```python
from build123d import *

# Parameters (mm, degrees)
EXTRUDE_1_DEPTH     = 4
EXTRUDE_START       = -2
SKETCH_2_R          = 0.75
EXTRUDE_2_DEPTH     = 1
SKETCH_3_R          = 0.75
CUT_EXTRUDE_1_DEPTH = 0.1
SKETCH_4_R          = 0.3
EXTRUDE_3_DEPTH     = 1.75


with BuildPart() as part:
    # 草图1 → 凸台-拉伸1 (new body)
    with BuildSketch(Plane.XY):
        with BuildLine():
            Line((0, 2), (9.3, 2))
            ThreePointArc((9.3, 2), (11.3, 0), (9.3, -2))
            Line((9.3, -2), (0, -2))
            ThreePointArc((0, -2), (-2, 0), (0, 2))
        make_face()
    extrude(amount=EXTRUDE_1_DEPTH)

    # 草图2 → 凸台-拉伸2 (add)
    with BuildSketch(Plane(origin=(0, 0, 0), x_dir=(-1, 0, 0), z_dir=(0, 0, -1)).offset(EXTRUDE_START)):
        with BuildLine():
            Line((-12.15, 2), (2.85, 2))
            ThreePointArc((2.85, 2), (4.85, 0), (2.85, -2))
            Line((2.85, -2), (-12.15, -2))
            ThreePointArc((-12.15, -2), (-14.15, 0), (-12.15, 2))
        make_face()
        with Locations((-12.7, 0)):
            Circle(SKETCH_2_R, mode=Mode.SUBTRACT)
        with Locations((3.4, 0)):
            Circle(SKETCH_2_R, mode=Mode.SUBTRACT)
    extrude(amount=-EXTRUDE_2_DEPTH)

    # 草图3 → 切除-拉伸1 (cut)
    with BuildSketch(Plane(origin=(0, 0, 0), x_dir=(-1, 0, 0), z_dir=(0, 0, -1))):
        with Locations((-6.05, 0)):
            Circle(SKETCH_3_R)
        with Locations((-3.25, 0)):
            Circle(SKETCH_3_R)
    extrude(amount=-CUT_EXTRUDE_1_DEPTH, mode=Mode.SUBTRACT)

    # 草图4 → 凸台-拉伸3 (add)
    with BuildSketch(Plane.XY.offset(4)):
        with Locations((3.25, 0)):
            Circle(SKETCH_4_R)
        with Locations((6.05, 0)):
            Circle(SKETCH_4_R)
    extrude(amount=EXTRUDE_3_DEPTH)


solid = part.part
```
Build history of the part. All positions in model axes, mm. A direction names the side the tool comes from. Round coordinates to 2 decimals unless told otherwise and drop trailing zeros. Write each loop counter-clockwise with the first axis right and the second up, starting at its lowest first coordinate (ties: lowest second). Pieces come first, ordered by that corner, then holes.
1) Pin check, flat tips, straight feed: pin 1 (1.2 mm diameter, centred on x = -3.5, y = -0.5, fed in from +Z); pin 2 (1.2 mm diameter, centred on x = 10.5, y = -1, fed in from +Z). Stop position of each tip, or through.
2) Mould opens along Y. For faces 5 (the flat face through (5, 0, 0)), 6 (the flat face through (6, 0, 0.1)), 7 (the cylindrical face through (13.45, 0.03, 2.49)), 8 (the cylindrical face through (-4.85, 0.04, 2.49)) say: +Y half, -Y half, draft (parallel to the pull), parting line (faces both ways), or undercut.
3) Drill centre lines: probe 1 along Y at (x, z) = (12.7, 2.65); probe 2 along Z at (x, y) = (7.25, 1.7); probe 3 along Z at (x, y) = (13, 1.6). Where is each one in solid material? Low to high.
4) Band-saw the part on C-C, the plane x = 12.5. List the corners of the cut face in (y, z), and give its area (3 significant figures).
5) Band-saw the part on A-A, the plane y = -1.6. List the corners of the cut face in (x, z).
6) Band-saw the part on B-B, the plane x = 3.25. List the corners of the cut face in (y, z), and give its area (3 significant figures).
7) 3-axis set-ups, long thin cutter, end or side, ignore diameter. For faces 1 (the cylindrical face through (-2, 0, 3.5)), 2 (the cylindrical face through (11.3, 0, 3.5)), 3 (the cylindrical face through (11.3, 0, 1)), 4 (the cylindrical face through (-2, 0, 1)): which of +Z, -Z, +X, -X, +Y, -Y reach the whole face in a straight line?
8) Band-saw the part on D-D, the plane y = 0. Give the number of separate pieces and of enclosed holes in the cut face, and give its area (3 significant figures).
Ans:
1. pin 1: stops at z = 3
1. pin 2: stops at z = 4
2. face 5: draft
2. face 6: undercut
2. face 7: undercut
2. face 8: parting line
3. probe 1: y = -1.92 to -0.75, 0.75 to 1.92
3. probe 2: z = 0 to 4
3. probe 3: z = 2 to 3
4. outline: (-1.97, 2) - (-0.72, 2) - (-0.72, 3) - (-1.97, 3) - close; (0.72, 2) - (1.97, 2) - (1.97, 3) - (0.72, 3) - close
4. area: 2.49 mm2
5. outline: (-4.05, 2) - (-1.2, 2) - (-1.2, 0) - (10.5, 0) - (10.5, 2) - (13.35, 2) - (13.35, 3) - (10.5, 3) - (10.5, 4) - (-1.2, 4) - (-1.2, 3) - (-4.05, 3) - close
6. outline: (-2, 0) - (-0.75, 0) - (-0.75, 0.1) - (0.75, 0.1) - (0.75, 0) - (2, 0) - (2, 4) - (0.3, 4) - (0.3, 5.75) - (-0.3, 5.75) - (-0.3, 4) - (-2, 4) - close
6. area: 16.9 mm2
7. face 1: +Z, -X
7. face 2: +Z, +X
7. face 3: -Z, +X
7. face 4: -Z, -X
8. separate pieces: 3
8. enclosed holes: 0
8. area: 57.7 mm2
